```python
from build123d import *
from build123d.topology import SkipClean

# Parameters (mm, degrees)
SKETCH_1_R      = 1.65
EXTRUDE_1_DEPTH = 1.6
SKETCH_2_W      = 22
SKETCH_2_H      = 6
EXTRUDE_2_DEPTH = 10
SKETCH_3_W      = 75.446569178
SKETCH_3_H      = 39.931008624
EXTRUDE_3_DEPTH = 36
SKETCH_4_W      = 8
SKETCH_4_H      = 20
EXTRUDE_4_DEPTH = 19
EXTRUDE_START   = 7
SKETCH_5_R      = 1.65
EXTRUDE_5_DEPTH = 7


with BuildPart() as part:
    # 草图1 → 凸台-拉伸1 (new body)
    with BuildSketch(Plane(origin=(0, 0, 0), x_dir=(1, 0, 0), z_dir=(0, 1, 0))):
        with BuildLine():
            Line((-44.5, -36), (44.5, -36))
            ThreePointArc((44.5, -36), (45.914213562, -35.414213562), (46.5, -34))
            Line((46.5, -34), (46.5, 34))
            ThreePointArc((46.5, 34), (45.914213562, 35.414213562), (44.5, 36))
            Line((44.5, 36), (-44.5, 36))
            ThreePointArc((-44.5, 36), (-45.914213562, 35.414213562), (-46.5, 34))
            Line((-46.5, 34), (-46.5, -34))
            ThreePointArc((-46.5, -34), (-45.914213562, -35.414213562), (-44.5, -36))
        make_face()
        with Locations(Location((-43, 32, 0), (0, 0, 270))):
            Circle(SKETCH_1_R, mode=Mode.SUBTRACT)
        with Locations(Location((43, 32, 0), (0, 0, 270))):
            Circle(SKETCH_1_R, mode=Mode.SUBTRACT)
        with Locations(Location((43, -32, 0), (0, 0, 270))):
            Circle(SKETCH_1_R, mode=Mode.SUBTRACT)
        with Locations(Location((-43, -32, 0), (0, 0, 270))):
            Circle(SKETCH_1_R, mode=Mode.SUBTRACT)
    extrude(amount=EXTRUDE_1_DEPTH)

    # 草图2 → 凸台-拉伸2 (add)
    with BuildSketch(Plane(origin=(0, 1.6, 0), x_dir=(1, 0, 0), z_dir=(0, 1, 0))):
        with Locations((-24.5, -30.5)):
            Rectangle(SKETCH_2_W, SKETCH_2_H)
        with Locations((25.5, -30.5)):
            Rectangle(SKETCH_2_W, SKETCH_2_H)
    extrude(amount=EXTRUDE_2_DEPTH)

    # 草图3 → 凸台-拉伸3 (add)
    with BuildSketch(Plane(origin=(0, 1.6, 0), x_dir=(1, 0, 0), z_dir=(0, 1, 0))):
        with Locations((-0.191976003, 15.406074241)):
            Rectangle(SKETCH_3_W, SKETCH_3_H)
    extrude(amount=EXTRUDE_3_DEPTH)

    # 草图4 → 凸台-拉伸4 (add)
    with BuildSketch(Plane(origin=(0, 1.6, 0), x_dir=(1, 0, 0), z_dir=(0, 1, 0))):
        with Locations((-42.5, 15)):
            Rectangle(SKETCH_4_W, SKETCH_4_H)
        with Locations((42.5, 15)):
            Rectangle(SKETCH_4_W, SKETCH_4_H)
    extrude(amount=EXTRUDE_4_DEPTH)

    # 草图5 → 凸台-拉伸5 (add)
    # profile 1 of 4: a face of its own
    with SkipClean():  # the faces are left unmerged after this step: merging them gives an invalid solid
        with BuildSketch(Plane.XZ.offset(EXTRUDE_START)):
            Polygon((39.940043573, -32), (41.470021787, -34.65), (44.529978213, -34.65), (46.059956427, -32), (44.529978213, -29.35), (41.470021787, -29.35), align=None)
            with Locations(Location((43, -32, 0), (0, 0, 270))):
                Circle(SKETCH_5_R, mode=Mode.SUBTRACT)
        # profile 2 of 4: a face of its own
        with BuildSketch(Plane.XZ.offset(EXTRUDE_START)):
            Polygon((-39.940043573, -32), (-41.470021787, -29.35), (-44.529978213, -29.35), (-46.059956427, -32), (-44.529978213, -34.65), (-41.470021787, -34.65), align=None)
            with Locations(Location((-43, -32, 0), (0, 0, 270))):
                Circle(SKETCH_5_R, mode=Mode.SUBTRACT)
        # profile 3 of 4: a face of its own
        with BuildSketch(Plane.XZ.offset(EXTRUDE_START)):
            Polygon((-39.940043573, 32), (-41.470021787, 34.65), (-44.529978213, 34.65), (-46.059956427, 32), (-44.529978213, 29.35), (-41.470021787, 29.35), align=None)
            with Locations(Location((-43, 32, 0), (0, 0, 270))):
                Circle(SKETCH_5_R, mode=Mode.SUBTRACT)
        # profile 4 of 4: a face of its own
        with BuildSketch(Plane.XZ.offset(EXTRUDE_START)):
            Polygon((39.940043573, 32), (41.470021787, 29.35), (44.529978213, 29.35), (46.059956427, 32), (44.529978213, 34.65), (41.470021787, 34.65), align=None)
            with Locations(Location((43, 32, 0), (0, 0, 270))):
                Circle(SKETCH_5_R, mode=Mode.SUBTRACT)
        extrude(amount=-EXTRUDE_5_DEPTH)


solid = part.part
```
For this review, take the finished solid that the model builds, in its own axes (mm). A direction names the side the tool comes from. Round coordinates to 2 decimals unless told otherwise and drop trailing zeros. Write each loop counter-clockwise with the first axis right and the second up, starting at its lowest first coordinate (ties: lowest second). Pieces come first, ordered by that corner, then holes.
1) For line 1 along Z through (x, y) = (-43, -1.75); line 2 along Z through (x, y) = (43, 1); line 3 along X through (y, z) = (1.15, 32), list the stretches that pass through material, from the lowest coordinate up.
Answer below:
line 1: z = -34.65 to -33.65, -30.35 to -29.35, 29.35 to 30.35, 33.65 to 34.65
line 2: z = -36 to -33.65, -30.35 to 30.35, 33.65 to 36
line 3: x = -46.5 to -44.65, -41.35 to 41.35, 44.65 to 46.5
2) Machinability: for faces 5 (the face through (-45.284, -3.549, -30.656)), 6 (the face through (-37.915, 19, -15)), 7 (the face through (40.694, -3.549, 30.694)), 8 (the face through (-43, 11, -25)), which of the approach directions +Z, -Z, +X, -X, +Y, -Y give a long, thin tool a straight path to every point of the face, cutting with its end or side? Answer none if there is none.
Answer below:
face 5: -X, -Y
face 6: +Z, -Z, +Y
face 7: -Y
face 8: -Z, -X, +Y
3) Take a section at D-D on x = 26.5. Give the boundary of the cut face in (y, z), then the cut area to 3 significant figures.
Answer below:
outline: (0, -36) - (1.6, -36) - (1.6, -35.37) - (37.6, -35.37) - (37.6, 4.56) - (1.6, 4.56) - (1.6, 27.5) - (11.6, 27.5) - (11.6, 33.5) - (1.6, 33.5) - (1.6, 36) - (0, 36) - close
area: 1,610 mm2
4) Take a section at C-C on z = -21. Give the boundary of the cut face in (x, y), then the cut area to 3 significant figures.
Answer below:
outline: (-46.5, 0) - (46.5, 0) - (46.5, 20.6) - (38.5, 20.6) - (38.5, 1.6) - (37.53, 1.6) - (37.53, 37.6) - (-37.92, 37.6) - (-37.92, 1.6) - (-38.5, 1.6) - (-38.5, 20.6) - (-46.5, 20.6) - close
area: 3,170 mm2
5) Insertion check: pin 1 Ø1 at (x, y) = (-36.5, 15.5) entering from -Z; pin 2 Ø10 at (x, y) = (15.5, 30) entering from +Z; pin 3 Ø4 at (x, y) = (42, 13) entering from +Z; pin 4 Ø2 at (x, z) = (43, 32) entering from -Y. Each pin has a flat end and moves straight along its axis. Give the tip position at first contact, or say it passes through.
Answer below:
pin 1: stops at z = -35.37
pin 2: stops at z = 4.56
pin 3: stops at z = -5
pin 4: passes through
6) Mouldability with a two-part tool opening along X and no side actions: class faces 1 (the face through (-43, -7, -34)), 2 (the face through (-40.694, -3.549, 33.306)), 3 (the face through (45.93, 0.79, -35.4)), 4 (the face through (-46.5, 8, -8)) as +X half, -X half, draft (parallel to the pull), parting line (faces both ways), or undercut.
Answer below:
face 1: draft
face 2: undercut
face 3: +X half
face 4: -X half
7) Take a section at B-B on x = -43. Give the boundary of the cut face in (y, z).
Answer below:
outline: (-7, -34.65) - (0, -34.65) - (0, -36) - (1.6, -36) - (1.6, -33.65) - (-7, -33.65) - close; (-7, -30.35) - (1.6, -30.35) - (1.6, -25) - (20.6, -25) - (20.6, -5) - (1.6, -5) - (1.6, 30.35) - (-7, 30.35) - (-7, 29.35) - (0, 29.35) - (0, -29.35) - (-7, -29.35) - close; (-7, 33.65) - (1.6, 33.65) - (1.6, 36) - (0, 36) - (0, 34.65) - (-7, 34.65) - close
8) Take a section at A-A on y = 3.5. Give the boundary of the cut face in (x, z).
Answer below:
outline: (-46.5, -25) - (-38.5, -25) - (-38.5, -5) - (-46.5, -5) - close; (-37.92, -35.37) - (37.53, -35.37) - (37.53, 4.56) - (-37.92, 4.56) - close; (-35.5, 27.5) - (-13.5, 27.5) - (-13.5, 33.5) - (-35.5, 33.5) - close; (14.5, 27.5) - (36.5, 27.5) - (36.5, 33.5) - (14.5, 33.5) - close; (38.5, -25) - (46.5, -25) - (46.5, -5) - (38.5, -5) - close
